The listing builds one solid part. Answer for the finished solid, in the listing's coordinates (mm). Coordinates: 2 decimals unless noted, no trailing zeros. Write each loop counter-clockwise with the first axis right and the second up, starting at its lowest first coordinate (ties: lowest second). Pieces come first, ordered by that corner, then holes.
Autodesk Inventor part; units mm, degrees
ref_plane "YZ Plane" through (0, 0, 0) normal (1, 0, 0) x (0, 1, 0)
ref_plane "XZ Plane" through (0, 0, 0) normal (0, 1, 0) x (-1, 0, 0)
ref_plane "XY Plane" through (0, 0, 0) normal (0, 0, 1) x (1, 0, 0)
sketch "Эскиз1" plane through (0, 0, 0) normal (1, 0, 0) x (0, 1, 0)
  line L0 (0, 0) -> (60, 0)
  line L1 (60, 0) -> (60, -178.77)
  line L2 (60, -178.77) -> (0, -178.77)
  line L3 (0, -178.77) -> (0, 0)
  dimension "d0" = 60
  dimension "d1" = 178.77
extrude "Выдавливание1" add sketch "Эскиз1" along normal blind 25
chamfer "Фаска1" distance 25 angle 45 2 edges at (25, 30, 0) (25, 30, -178.77)
sketch "Эскиз2" plane through (0, 60, 0) normal (0, 1, 0) x (1, 0, 0)
  line L0 (25, 153.77) -> (3.5, 175.27)
  arc A0 (10, 168.77) -> (10, 10) centre (320.0989, 89.385) ccw
  line L1 (0, 0) -> (0, 178.77)
  line L2 (0, 89.385) -> (124.8295, 89.385)
  line L3 (25, 25) -> (0, 0)
  arc A1 (25, 153.77) -> (25, 25) centre (320.0989, 89.385) ccw
  line L4 (0, 178.77) -> (25, 153.77)
  line L5 (0, 0) -> (0, 178.77)
  line L6 (25, 25) -> (0, 0)
  line L7 (25, 153.77) -> (25, 25)
  line L8 (10, 10) -> (0, 0)
  line L9 (0, 0) -> (0, 89.385)
  line L10 (0, 89.385) -> (0, 178.77)
  line L11 (10, 168.77) -> (0, 178.77)
  line L12 (25, 153.77) -> (25, 25)
  point P0 (7, 178.77)
  dimension "d7" = 10
extrude "Выдавливание2" cut sketch "Эскиз2" against normal blind 60 contours A0 L1 L4 L0 | A0 L3 L1
properties part number "Short" material "Красное дерево"
Q1. Find the intervals of material crossed by probe 1 along X at (y, z) = (15, -81.5); probe 2 along X at (y, z) = (55.5, -149); probe 3 along Z at (x, y) = (19.75, 10), in increasing order.
Answers below:
probe 1: x = 0.1 to 25
probe 2: x = 5.6 to 25
probe 3: z = -159.02 to -19.75
Q2. The part is cut by section B-B, the plane z = -134.5. Write down the section's boundary in (x, y), then the cut area to 3 significant figures.
Answers below:
outline: (3.2, 0) - (25, 0) - (25, 60) - (3.2, 60) - close
area: 1,310 mm2
Q3. Given pin 1 (1.5 mm diameter, centred on y = 27.5, z = -148.5, fed in from -X); pin 2 (3 mm diameter, centred on x = 15, y = 32, fed in from -Z); pin 3 (1 mm diameter, centred on x = 12.5, y = 22.5, fed in from -Z), each flat-ended and moving along its own axis, determine where each tip first touches the part or whether it passes through.
Answers below:
pin 1: stops at x = 5.37
pin 2: stops at z = -165.27
pin 3: stops at z = -166.77
